Could you check a few things on this model? Use its own coordinates, in mm. A direction names the side the tool comes from. Give positions to 0.01 mm unless a question says otherwise; leave off trailing zeros. Order: outer loops, then holes, each group sorted by start corner. A loop starts at its lowest first (then second) coordinate and runs counter-clockwise, first axis right, second up. Notation, with made-up numbers: (5.25, 71) -> (18.25, 71) arc R18 cw to (18.25, 77) -> close; hole circle Ø6 at (89, -38.5). An arc over 180 degrees is marked (long way). Use one line per item in the form item = value. Start each with the question number.
from build123d import *
from build123d.topology import SkipClean

# Parameters (mm, degrees)
SKETCH2_R           = 13.335
SKETCH2_R_2         = 12.7
BOSS_EXTRUDE1_DEPTH = 0.508
BOSS_EXTRUDE2_START = 1.27
SKETCH3_R           = 15.24
SKETCH3_R_2         = 13.335
BOSS_EXTRUDE2_DEPTH = 1.27
CUT_EXTRUDE1_DEPTH  = 97.736659463
BOSS_EXTRUDE3_DEPTH = 0.508


with BuildPart() as part:
    # Sketch2 → Boss-Extrude1 (new body)
    with BuildSketch(Plane.XY):
        with BuildLine():
            Line((12.7, 0), (25.4, 0))
            ThreePointArc((25.4, 0), (34.380256121, 3.719743879), (38.1, 12.7))
            Line((38.1, 12.7), (38.1, 76.2))
            ThreePointArc((38.1, 76.2), (34.380256121, 85.180256121), (25.4, 88.9))
            Line((25.4, 88.9), (12.7, 88.9))
            ThreePointArc((12.7, 88.9), (3.719743879, 85.180256121), (0, 76.2))
            Line((0, 76.2), (0, 12.7))
            ThreePointArc((0, 12.7), (3.719743879, 3.719743879), (12.7, 0))
        make_face()
        with Locations((19.05, 69.85)):
            Circle(SKETCH2_R, mode=Mode.SUBTRACT)
        with Locations((19.05, 19.05)):
            Circle(SKETCH2_R_2, mode=Mode.SUBTRACT)
    extrude(amount=BOSS_EXTRUDE1_DEPTH)

    # Sketch3 → Boss-Extrude2 (add)
    with SkipClean():  # the faces are left unmerged after this step: merging them gives an invalid solid
        with BuildSketch(Plane(origin=(0, 0, 0), x_dir=(-1, 0, 0), z_dir=(0, 0, -1)).offset(BOSS_EXTRUDE2_START)):
            with Locations((-19.05, 69.85)):
                Circle(SKETCH3_R)
            with Locations((-19.05, 69.85)):
                Circle(SKETCH3_R_2, mode=Mode.SUBTRACT)
        boss_extrude2 = extrude(amount=-BOSS_EXTRUDE2_DEPTH)

    # Mirror1: Boss-Extrude2 across plane
    add(boss_extrude2.mirror(Plane(origin=(0, 0, 0.254), x_dir=(1, 0, 0), z_dir=(0, 0, -1))))

    # Sketch4 → Cut-Extrude1 (cut, through all)
    with BuildSketch(Plane(origin=(0, 0, 0), x_dir=(-1, 0, 0), z_dir=(0, 0, -1))):
        with BuildLine():
            Line((-31.75, 29.058935454), (-31.75, 59.841064546))
            ThreePointArc((-31.75, 59.841064546), (-19.05, 53.025291513), (-6.35, 59.841064546))
            Line((-6.35, 59.841064546), (-6.35, 29.058935454))
            ThreePointArc((-6.35, 29.058935454), (-19.05, 34.319447696), (-31.75, 29.058935454))
        make_face()
    extrude(amount=-CUT_EXTRUDE1_DEPTH, mode=Mode.SUBTRACT)

    # Sketch5 → Boss-Extrude3 (add)
    with BuildSketch(Plane(origin=(0, 0, 0), x_dir=(-1, 0, 0), z_dir=(0, 0, -1))):
        Polygon((-20.32, 53.025291513), (-20.32, 34.319447696), (-20.32, 34.162691866), (-17.78, 34.162691866), (-17.78, 34.23115412), (-17.78, 34.319447696), (-17.78, 53.025291513), (-17.78, 53.171866838), (-20.32, 53.171866838), align=None)
    extrude(amount=-BOSS_EXTRUDE3_DEPTH)


solid = part.part
(1) Please list where these lines run through material, in increasing order: probe 1 along Y at (x, z) = (19.05, 0.45) (3 decimals); probe 2 along Y at (x, z) = (19.05, 1.25) (3 decimals); probe 3 along X at (y, z) = (69.85, 0.2) (3 decimals).
(2) Imagine slicing it at B-B (y = 39.5). Write out the boundary of the cut face in (x, z).
(3) We'd pull the mould along Y, two halves only. Please class faces 4 (the cylindrical face through (11.37, 55.1, 0.25)), 5 (the cylindrical face through (34.28, 3.62, 0.25)), 6 (the cylindrical face through (3.82, 85.28, 0.25)): pulls with the +Y half, pulls with the -Y half, needs draft (parallel to the pull), parting line crosses it, or undercut.
(4) I'm going to push flat-ended pins straight in: pin 1 Ø16 at (x, y) = (19.05, 69.85) entering from -Z; pin 2 Ø4 at (x, y) = (31, 46.5) entering from -Z; pin 3 Ø1.5 at (x, z) = (11.5, 0.5) entering from -Y. Where does each tip first touch, or does it pass through?
(5) Imagine slicing it at A-A (x = 19.05). Write out the boundary of the cut face in (y, z) (3 decimals).
(6) Which directions (+Z, -Z, +X, -X, +Y, -Y) give clear straight access to the entire face, cutting with the end or side of a thin tool? Please do faces 1 (the flat face through (19, 45, 0)), 2 (the cylindrical face through (30.782, 14.186, 0.25)), 3 (the flat face through (19, 45, 0.508)).
(7) Imagine slicing it at D-D (x = 23). Write out the boundary of the cut face in (y, z).
(8) Imagine slicing it at C-C (y = 19.05). Write out the boundary of the cut face in (x, z).
Calculated:
q1.probe_1 = 0 to 6.35, 31.75 to 56.515, 83.185 to 88.9
q1.probe_2 = 54.61 to 56.515, 83.185 to 85.09
q1.probe_3 = 0 to 5.715, 32.385 to 38.1
q2.outline = (0, 0) -> (6.35, 0) -> (6.35, 0.51) -> (0, 0.51) -> close; (17.78, 0) -> (20.32, 0) -> (20.32, 0.51) -> (17.78, 0.51) -> close; (31.75, 0) -> (38.1, 0) -> (38.1, 0.51) -> (31.75, 0.51) -> close
q3.face_4 = undercut
q3.face_5 = pulls with the -Y half
q3.face_6 = pulls with the +Y half
q4.pin_1 = through
q4.pin_2 = 0
q4.pin_3 = 0.01
q5.outline = (0, 0) -> (6.35, 0) -> (6.35, 0.508) -> (0, 0.508) -> close; (31.75, 0) -> (54.61, 0) -> (54.61, -1.27) -> (56.515, -1.27) -> (56.515, 1.778) -> (54.61, 1.778) -> (54.61, 0.508) -> (31.75, 0.508) -> close; (83.185, -1.27) -> (85.09, -1.27) -> (85.09, 0) -> (88.9, 0) -> (88.9, 0.508) -> (85.09, 0.508) -> (85.09, 1.778) -> (83.185, 1.778) -> close
q6.face_1 = -Z
q6.face_2 = +Z, -Z
q6.face_3 = +Z
q7.outline = (0, 0) -> (6.98, 0) -> (6.98, 0.51) -> (0, 0.51) -> close; (31.12, 0) -> (33.88, 0) -> (33.88, 0.51) -> (31.12, 0.51) -> close; (53.55, 0) -> (55.13, 0) -> (55.13, -1.27) -> (57.11, -1.27) -> (57.11, 1.78) -> (55.13, 1.78) -> (55.13, 0.51) -> (53.55, 0.51) -> close; (82.59, -1.27) -> (84.57, -1.27) -> (84.57, 0) -> (88.9, 0) -> (88.9, 0.51) -> (84.57, 0.51) -> (84.57, 1.78) -> (82.59, 1.78) -> close
q8.outline = (0, 0) -> (6.35, 0) -> (6.35, 0.51) -> (0, 0.51) -> close; (31.75, 0) -> (38.1, 0) -> (38.1, 0.51) -> (31.75, 0.51) -> close
